```python
from build123d import *

# Parameters (mm, degrees)
BOSS_EXTRUDE1_DEPTH = 50
SKETCH3_W           = 3.3
SKETCH3_H           = 1
BOSS_EXTRUDE2_DEPTH = 13
BOSS_EXTRUDE3_DEPTH = 53.5
SKETCH6_W           = 4.8
SKETCH6_H           = 40
BOSS_EXTRUDE4_DEPTH = 5
CHAMFER1_START      = -14
CHAMFER1_OUTLINE_W  = 52
CHAMFER1_OUTLINE_H  = 13
CHAMFER1_DEPTH      = 3.182909169
CHAMFER2_SIZE       = 3


with BuildPart() as part:
    # Sketch2 → Boss-Extrude1 (new body)
    with BuildSketch(Plane(origin=(0, 0, 0), x_dir=(1, 0, 0), z_dir=(0, 1, 0))):
        Polygon((-1.7, -2), (-1.7, -15), (-5.7, -15), (-5.7, -2), (-9, -2), (-9, -15), (-13, -15), (-13, 2.680601608), align=None)
    extrude(amount=BOSS_EXTRUDE1_DEPTH)

    # Sketch3 → Boss-Extrude2 (add)
    with BuildSketch(Plane.XY.offset(2)):
        with Locations((-7.35, 0.5)):
            Rectangle(SKETCH3_W, SKETCH3_H)
    extrude(amount=BOSS_EXTRUDE2_DEPTH)

    # Sketch5 → Boss-Extrude3 (add)
    with BuildSketch(Plane.XY.offset(15)):
        Polygon((-13, 0), (-1.7, 0), (-1.7, 14), (-5.7, 14), (-5.7, 1), (-9, 1), (-9, 14), (-13, 14), align=None)
    extrude(amount=BOSS_EXTRUDE3_DEPTH)

    # Sketch6 → Boss-Extrude4 (add)
    with BuildSketch(Plane(origin=(0, 0, 0), x_dir=(-1, 0, 0), z_dir=(0, -1, 0))):
        with Locations((7.35, -35)):
            Rectangle(SKETCH6_W, SKETCH6_H)
    extrude(amount=BOSS_EXTRUDE4_DEPTH)

    # Mirror1: part across plane


with BuildPart() as part_1:
    add(part.part)
    add(part.part.mirror(Plane(origin=(-0.956063716, 0, 2.308147732), x_dir=(0.9238798691632129, 0, 0.38268261961443256), z_dir=(0.3826826196144326, 0, -0.9238798691632131))))

    # Chamfer1: read off the stored shape, not the designer's step
    # Chamfer1 outline → Chamfer1 (cut)
    with BuildSketch(Plane(origin=(0, 0, 0), x_dir=(0, 1, 0), z_dir=(0.9238798691632129, 0, 0.38268261961443295)).offset(CHAMFER1_START)):
        with Locations((25, 2.5)):
            Rectangle(CHAMFER1_OUTLINE_W, CHAMFER1_OUTLINE_H)
    extrude(amount=CHAMFER1_DEPTH, mode=Mode.SUBTRACT)

    # Chamfer2
    chamfer2_edges = [part_1.edges().sort_by_distance(p)[0] for p in [
        (-13, 32, 15),
        (-13, 14, 41.75),
        (-0.497948704, 32, -15.182696898),
        (18.417124413, 14, -34.097836574),
    ]]
    chamfer(chamfer2_edges, length=CHAMFER2_SIZE)


solid = part_1.part
```
Verification items for the finished model (mm, model axes). A direction names the side the tool comes from. Coordinates: 2 decimals unless noted, no trailing zeros. Loops run counter-clockwise (first coordinate to the right, second up) from the corner with the lowest first, then second, coordinate; pieces in that order, holes last. Notation, with made-up numbers: (-22.75, -37.5) -> (2.25, -37.5) arc R21 cw to (2.25, -13.5) -> close; hole circle Ø3 at (13.25, 73). An arc over 180 degrees is marked (long way). Answer in a Markdown table with one row per item. Add a question column.
1. Section check C-C, the plane x = 12. Enter the section's corners in (y, z), then the cut area to 3 significant figures.
2. Access from +Z, -Z, +X, -X, +Y, -Y to the whole of each face (thin tool, end or side, straight path). Record for faces 1 (the face through (-7, -2, 15)), 2 (the face through (-4, 32, 15)), 3 (the face through (16.14, -2.465, -27.225)), 4 (the face through (-1.7, 13.5, 27.4)).
3. Depth check by flat-ended pin: P1, Ø3.5, axis at x = -0.5, y = 37.5, coming from the -Z side; P2, Ø8, axis at y = 32.5, z = 6.5, coming from the +X side; P3, Ø8, axis at y = 7.5, z = 2.5, coming from the +X side. Enter the tip coordinate at first touch or a pass-through.
4. Material ranges on probe 1 along Y at (x, z) = (-10, 8); probe 2 along Y at (x, z) = (7, -16.5); probe 3 along Z at (x, y) = (14, 3.5), recorded low to high. Write a range as [from, to].
5. Section check B-B, the plane y = 34. Enter the section's corners in (x, z).
6. Draft check along Z on faces 5 (the face through (-11, 30, 14)), 6 (the face through (17, -5, -25)), 7 (the face through (5.871, 8.824, -15.895)), 8 (the face through (-5.7, 25.2, -2)). Enter one of: +Z half, -Z half, draft (parallel to the pull), parting line (faces both ways), or undercut.
7. Section check A-A, the plane z = 22.5. Enter the section's corners in (x, y).
8. Section check D-D, the plane y = 7. Enter the section's corners in (x, z), then the cut area to 4 significant figures.
Derived:
| question | item | result |
|---|---|---|
| 1 | outline | (-5, -23.08) -> (0, -23.08) -> (0, -27.68) -> (11, -27.68) -> (14, -23.44) -> (14, -22.02) -> (1, -22.02) -> (1, -17.36) -> (14, -17.36) -> (14, -11.7) -> (0, -11.7) -> (0, -16.3) -> (-5, -16.3) -> close |
| 1 | area | 191 mm² |
| 2 | face 1 | -Z, +X, -X, -Y |
| 2 | face 2 | +Z, +X, -X, +Y |
| 2 | face 3 | -Z, -X, -Y |
| 2 | face 4 | +Z, +X, +Y, -Y |
| 3 | P1 | stops at z = -13.06 |
| 3 | P2 | stops at x = -1.7 |
| 3 | P3 | stops at x = 1.8 |
| 4 | probe 1 | y = [0, 50] |
| 4 | probe 2 | y = [-5, 1] |
| 4 | probe 3 | z = [-29.68, -24.02], [-19.36, -13.7] |
| 5 | outline | (-13, 3.12) -> (-8.9, -6.78) -> (-2.62, -13.06) -> (1.62, -13.06) -> (2.33, -12.35) -> (-6.86, -3.16) -> (-4.53, -0.83) -> (4.66, -10.02) -> (7.49, -7.19) -> (-1.7, 2) -> (-1.7, 15) -> (-5.7, 15) -> (-5.7, 2) -> (-9, 2) -> (-9, 15) -> (-10, 15) -> (-13, 12) -> close |
| 6 | face 5 | +Z half |
| 6 | face 6 | draft |
| 6 | face 7 | undercut |
| 6 | face 8 | undercut |
| 7 | outline | (-13, 0) -> (-9.75, 0) -> (-9.75, -5) -> (-4.95, -5) -> (-4.95, 0) -> (-1.7, 0) -> (-1.7, 14) -> (-5.7, 14) -> (-5.7, 1) -> (-9, 1) -> (-9, 14) -> (-10, 14) -> (-13, 11) -> close |
| 8 | outline | (-13, 3.12) -> (-8.9, -6.78) -> (37.33, -53.01) -> (40.16, -50.18) -> (-6.86, -3.16) -> (-4.53, -0.83) -> (42.49, -47.85) -> (45.32, -45.02) -> (-1.7, 2) -> (-1.7, 68.5) -> (-5.7, 68.5) -> (-5.7, 2) -> (-9, 2) -> (-9, 68.5) -> (-13, 68.5) -> close |
| 8 | area | 1,105 mm² |
